Part model, mm, in its own coordinate system. A direction names the side the tool comes from. Give positions to 0.01 mm unless a question says otherwise; leave off trailing zeros. Order: outer loops, then holes, each group sorted by start corner. A loop starts at its lowest first (then second) coordinate and runs counter-clockwise, first axis right, second up. Notation, with made-up numbers: M 37.5,48.25 L 90.5,48.25 A16 cw 90.5,62.25 Z; hole C 52,-27.5 d10. An arc over 180 degrees is marked long. One line per question, with ' | ' between items.
```python
from build123d import *

# Parameters (mm, degrees)
SKETCH2_W           = 27.94
SKETCH2_H           = 25.4
SKETCH2_W_2         = 25.908
SKETCH2_H_2         = 24.13
BOSS_EXTRUDE1_DEPTH = 2.032
SKETCH3_W           = 27.94
SKETCH3_H           = 25.4
BOSS_EXTRUDE2_DEPTH = 2.54
SKETCH4_R           = 13.87475
BOSS_EXTRUDE3_DEPTH = 28.175
FILLET1_R           = 2.54


with BuildPart() as part:
    # Sketch2 → Boss-Extrude1 (new body)
    with BuildSketch(Plane.XY):
        Rectangle(SKETCH2_W, SKETCH2_H)
        Rectangle(SKETCH2_W_2, SKETCH2_H_2, mode=Mode.SUBTRACT)
    extrude(amount=BOSS_EXTRUDE1_DEPTH)

    # Sketch3 → Boss-Extrude2 (add)
    with BuildSketch(Plane(origin=(0, 0, 0), x_dir=(-1, 0, 0), z_dir=(0, 0, -1))):
        Rectangle(SKETCH3_W, SKETCH3_H)
    extrude(amount=BOSS_EXTRUDE2_DEPTH)

    # Sketch4 → Boss-Extrude3 (add)
    with BuildSketch(Plane(origin=(0, 0, -2.54), x_dir=(-1, 0, 0), z_dir=(0, 0, -1))):
        with Locations(Location((0, 0, 0), (0, 0, 246.252892173))):
            Circle(SKETCH4_R)
    extrude(amount=BOSS_EXTRUDE3_DEPTH)

    # Fillet1
    fillet1_edges = [part.edges().sort_by_distance(p)[0] for p in [
        (-13.97, 12.7, -0.254),
        (13.97, 12.7, -0.254),
        (13.97, -12.7, -0.254),
        (-13.97, -12.7, -0.254),
    ]]
    fillet(fillet1_edges, radius=FILLET1_R)


solid = part.part
```
1. Slice it at B-B on y = 0. Give the cut face in (x, z) (3 decimals), then the cut area to 3 significant figures.
Worked out:
outline: M -13.97,-2.54 L -13.875,-2.54 L -13.875,-30.715 L 13.875,-30.715 L 13.875,-2.54 L 13.97,-2.54 L 13.97,2.032 L 12.954,2.032 L 12.954,0 L -12.954,0 L -12.954,2.032 L -13.97,2.032 Z | area: 857 mm2
2. Drop flat-ended pins along their axis: pin 1 (3 mm diameter, centred on x = 9, z = -26, fed in from -Y); pin 2 (8 mm diameter, centred on x = 3.5, y = -11, fed in from +Z); pin 3 (1 mm diameter, centred on x = 4, z = 1, fed in from -Y); pin 4 (3 mm diameter, centred on x = 5.5, z = -15.5, fed in from +Y). Give the stop position or say it passes through.
Worked out:
pin 1: stops at y = -11.67 | pin 2: stops at z = 2.03 | pin 3: stops at y = -12.7 | pin 4: stops at y = 13.29
3. Probe L1, parallel to Z at x = 6.5, y = 5.75 (3 decimals); L2, parallel to Y at x = 0.5, z = -26.5; L3, parallel to Y at x = -3, z = -2.5. List the from-to ranges inside material, lowest first. Write a range as from..to.
Worked out:
L1: z = -30.715..0 | L2: y = -13.87..13.87 | L3: y = -12.7..12.7
4. Mould opens along X. For faces 4 (the cylindrical face through (-13.206, 11.976, -0.222)), 5 (the cylindrical face through (13.206, 11.976, -0.222)), 6 (the flat face through (-0.1, 12.3, 2.032)), 7 (the flat face through (0, 0, 0)) say: released by +X, released by -X, zero draft, split by the parting line, or undercut.
Worked out:
face 4: released by -X | face 5: released by +X | face 6: zero draft | face 7: undercut
5. Slice it at A-A on z = 0.5. Give the cut face in (x, y) (3 decimals), then the cut area to 3 significant figures.
Worked out:
outline: M -13.97,-10.16 A2.54 ccw -11.43,-12.7 L 11.43,-12.7 A2.54 ccw 13.97,-10.16 L 13.97,10.16 A2.54 ccw 11.43,12.7 L -11.43,12.7 A2.54 ccw -13.97,10.16 Z; hole M -12.954,-12.065 L 12.954,-12.065 L 12.954,12.065 L -12.954,12.065 Z | area: 79.0 mm2
6. Slice it at C-C on x = 0. Give the cut face in (y, z) (3 decimals).
Worked out:
outline: M -13.875,-30.715 L 13.875,-30.715 L 13.875,-2.54 L 12.7,-2.54 L 12.7,2.032 L 12.065,2.032 L 12.065,0 L -12.065,0 L -12.065,2.032 L -12.7,2.032 L -12.7,-2.54 L -13.875,-2.54 Z
7. Slice it at D-D on z = -20. Give the cut face in (x, y), then the cut area to 3 significant figures.
Worked out:
outline: C 0,0 d27.75 | area: 605 mm2
8. Tool access for faces 1 (the flat face through (13.8, -2.8, -2.54)), 2 (the flat face through (-12.954, 0, 1)), 3 (the flat face through (0, 12.7, 0)): list every direction of +Z, -Z, +X, -X, +Y, -Y with a clear straight run to the whole face (end or side of a thin tool).
Worked out:
face 1: -Z, +X | face 2: +Z | face 3: +Z, +X, -X, +Y
